Job drawing, mm, ordinate dimensions from the low corner. One solid piece. A direction names the side the tool comes from. Round coordinates to 2 decimals unless told otherwise and drop trailing zeros. Loops run counter-clockwise (first coordinate to the right, second up) from the corner with the lowest first, then second, coordinate; pieces in that order, holes last.
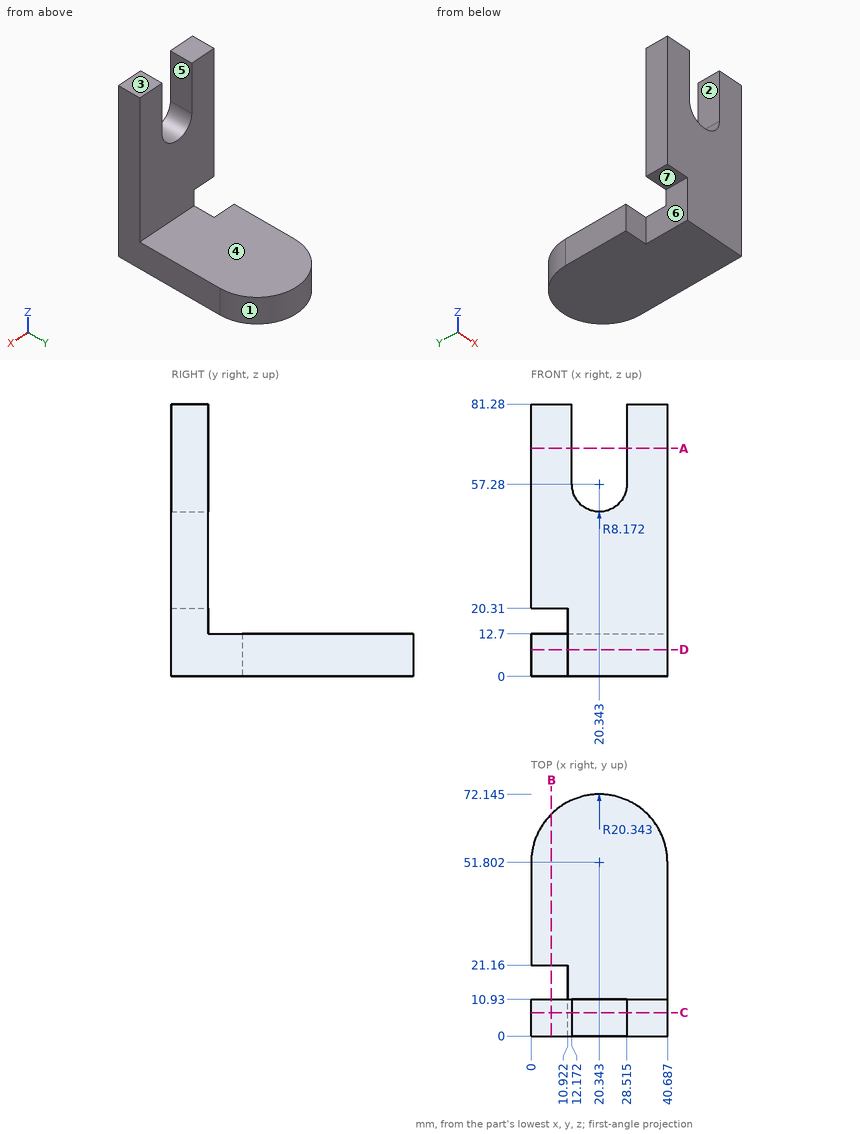
1) Tool access for the marked faces 4, 5, 6 and 7: list every direction of +Z, -Z, +X, -X, +Y, -Y with a clear straight run to the whole face (end or side of a thin tool).
Values:
face 4: +Z, +X, -X, +Y
face 5: +Z, +Y, -Y
face 6: -Z, -X, -Y
face 7: -Z, -X, +Y, -Y
2) Wall check: line 1 along X through (y, z) = (9.5, 61) (1 decimal); line 2 along Z through (x, y) = (6.5, 51); line 3 along Y through (x, z) = (23, 23). Give the ranges that are in metal, low to high.
Values:
line 1: x = 0 to 12.2, 28.5 to 40.7
line 2: z = 0 to 12.7
line 3: y = 0 to 10.93
3) Slice it at D-D, the plane z = 8. Give the cut face in (x, y).
Values:
outline: (0, 21.16) - (10.92, 21.16) - (10.92, 0) - (40.69, 0) - (40.69, 51.8) arc R20.34 ccw to (0, 51.8) - close
4) Mould opens along X. For the marked faces 1, 2 and 3 say: released by +X, released by -X, zero draft, split by the parting line, or undercut.
Values:
face 1: split by the parting line
face 2: undercut
face 3: zero draft
5) Slice it at A-A, the plane z = 68. Give the cut face in (x, y) (1 decimal), then the cut area to 3 significant figures.
Values:
outline: (0, 0) - (12.2, 0) - (12.2, 10.9) - (0, 10.9) - close; (28.5, 0) - (40.7, 0) - (40.7, 10.9) - (28.5, 10.9) - close
area: 266 mm2
6) Slice it at B-B, the plane x = 6. Give the cut face in (y, z), then the cut area to 3 significant figures.
Values:
outline: (0, 20.31) - (10.93, 20.31) - (10.93, 81.28) - (0, 81.28) - close; (21.16, 0) - (66.23, 0) - (66.23, 12.7) - (21.16, 12.7) - close
area: 1,240 mm2
7) Slice it at C-C, the plane y = 7. Give the cut face in (x, z) (1 decimal), then the cut area to 3 significant figures.
Values:
outline: (0, 20.3) - (10.9, 20.3) - (10.9, 0) - (40.7, 0) - (40.7, 81.3) - (28.5, 81.3) - (28.5, 57.3) arc R8.2 cw to (12.2, 57.3) - (12.2, 81.3) - (0, 81.3) - close
area: 2,590 mm2
8) Drop flat-ended pins along their axis: pin 1 Ø16 at (y, z) = (8, 12) entering from -X; pin 2 Ø3.5 at (x, y) = (7.5, 4) entering from -Z; pin 3 Ø3.5 at (x, z) = (6, 4.5) entering from -Y. Give the stop position or say it passes through.
Values:
pin 1: stops at x = 10.92
pin 2: stops at z = 20.31
pin 3: stops at y = 21.16
